Check sheet for the modelled part. Datum: model origin and axes. Units: mm. A direction names the side the tool comes from. Round coordinates to 2 decimals unless told otherwise and drop trailing zeros. Loops run counter-clockwise (first coordinate to the right, second up) from the corner with the lowest first, then second, coordinate; pieces in that order, holes last. Notation, with made-up numbers: (3.5, 63) - (27.5, 63) arc R27 cw to (27.5, 81) - close; hole circle Ø8 at (10.5, 46.5). An arc over 180 degrees is marked (long way). Put each result on its own line as item: value. Start each with the question number.
```python
from build123d import *

# Parameters (mm, degrees)
SKETCH1_W                                      = 45
SKETCH1_H                                      = 14
BOSS_EXTRUDE1_DEPTH                            = 12.7
SKETCH2_W                                      = 45
SKETCH2_H                                      = 10
CUT_EXTRUDE1_DEPTH                             = 10.7
CSK_FOR_M2_FLAT_HEAD_MACHINE_SCREW1_AT_2_COUNT = 2
CSK_FOR_M2_FLAT_HEAD_MACHINE_SCREW1_AT_2_PITCH = 34.2
CUT_EXTRUDE2_DEPTH                             = 30.386051113
CUT_EXTRUDE2_DEPTH_BACK                        = 30.386051113
SKETCH5_R                                      = 2.125


with BuildPart() as part:
    # Sketch1 → Boss-Extrude1 (new body)
    with BuildSketch(Plane.XY):
        Rectangle(SKETCH1_W, SKETCH1_H)
    extrude(amount=BOSS_EXTRUDE1_DEPTH)

    # Sketch2 → Cut-Extrude1 (cut)
    with BuildSketch(Plane.XY.offset(12.7)):
        Rectangle(SKETCH2_W, SKETCH2_H)
    extrude(amount=-CUT_EXTRUDE1_DEPTH, mode=Mode.SUBTRACT)

    # Sketch3 → CSK for M2 Flat Head Machine Screw1 (revolve, cut)
    with BuildSketch(Plane(origin=(-17.1, 0, 2), x_dir=(0, -1, 0), z_dir=(1, 0, 0))):
        Polygon((0, 0), (0, 2), (1.2, 2), (1.2, 1), (2.2, 0), align=None)
    csk_for_m2_flat_head_machine_screw1 = revolve(axis=Axis((-17.1, 0, 8.35), (0, 0, -1)), mode=Mode.SUBTRACT)

    # CSK for M2 Flat Head Machine Screw1 at 2: CSK for M2 Flat Head Machine Screw1 ×2
    with Locations(*[(i * CSK_FOR_M2_FLAT_HEAD_MACHINE_SCREW1_AT_2_PITCH, 0, 0) for i in range(1, CSK_FOR_M2_FLAT_HEAD_MACHINE_SCREW1_AT_2_COUNT)]):
        add(csk_for_m2_flat_head_machine_screw1, mode=Mode.SUBTRACT)

    # Sketch5 → Cut-Extrude2 (cut, two sides: drawn at the far end of the back side and taken through both)
    with BuildSketch(Plane(origin=(0, 7, 0), x_dir=(1, 0, 0), z_dir=(0, 1, 0)).offset(-CUT_EXTRUDE2_DEPTH_BACK)):
        with Locations(Location((0, -9.525, 0), (0, 0, 270))):
            Circle(SKETCH5_R)
    extrude(amount=CUT_EXTRUDE2_DEPTH + CUT_EXTRUDE2_DEPTH_BACK, mode=Mode.SUBTRACT)


solid = part.part
```
Q1. Cross-section at D-D on x = 0. Enter the section's corners in (y, z).
Q2. Set-up check for faces 4 (the face through (0, -6, 12.7)), 5 (the face through (0, 5, 6)): record each of +Z, -Z, +X, -X, +Y, -Y from which the full face is reachable in a straight line by a thin tool's end or side.
Q3. Cross-section at B-B on y = 0. Enter the section's corners in (x, z), and give its area (3 significant figures).
Q4. Cross-section at A-A on x = 17.1. Enter the section's corners in (y, z), and give its area (3 significant figures).
Q5. Material ranges on line 1 (X direction, y = 0, z = 0.4); line 2 (Y direction, x = -19.5, z = 11); line 3 (Y direction, x = -17.1, z = 0.2), recorded low to high. Write a range as from..to.
Q6. Cross-section at C-C on z = 6.5. Enter the section's corners in (x, y).
Q7. Draft check along Y on faces 1 (the face through (0, -7, 6)), 2 (the face through (0, -5, 6)), 3 (the face through (0, 0, 0)). Enter one of: +Y half, -Y half, draft (parallel to the pull), parting line (faces both ways), or undercut.
Answer list:
1. outline: (-7, 0) - (7, 0) - (7, 7.4) - (5, 7.4) - (5, 2) - (-5, 2) - (-5, 7.4) - (-7, 7.4) - close; (-7, 11.65) - (-5, 11.65) - (-5, 12.7) - (-7, 12.7) - close; (5, 11.65) - (7, 11.65) - (7, 12.7) - (5, 12.7) - close
2. face 4: +Z, +X, -X, +Y, -Y
2. face 5: +Z, +X, -X
3. outline: (-22.5, 0) - (-18.3, 0) - (-18.3, 1) - (-19.3, 2) - (-22.5, 2) - close; (-15.9, 0) - (15.9, 0) - (15.9, 1) - (14.9, 2) - (-14.9, 2) - (-15.9, 1) - close; (18.3, 0) - (22.5, 0) - (22.5, 2) - (19.3, 2) - (18.3, 1) - close
3. area: 78.4 mm2
4. outline: (-7, 0) - (-1.2, 0) - (-1.2, 1) - (-2.2, 2) - (-5, 2) - (-5, 12.7) - (-7, 12.7) - close; (1.2, 0) - (7, 0) - (7, 12.7) - (5, 12.7) - (5, 2) - (2.2, 2) - (1.2, 1) - close
4. area: 65.0 mm2
5. line 1: x = -22.5..-18.3, -15.9..15.9, 18.3..22.5
5. line 2: y = -7..-5, 5..7
5. line 3: y = -7..-1.2, 1.2..7
6. outline: (-22.5, -7) - (22.5, -7) - (22.5, -5) - (-22.5, -5) - close; (-22.5, 5) - (22.5, 5) - (22.5, 7) - (-22.5, 7) - close
7. face 1: -Y half
7. face 2: undercut
7. face 3: draft
